```python
from build123d import *

# Parameters (mm, degrees)
SKETCH1_R                = 14.5
BOSS_EXTRUDE1_DEPTH      = 4
BOSS_EXTRUDE2_DEPTH      = 2
BOSS_EXTRUDE2_DEPTH_BACK = 125
SKETCH2_R                = 5
SKETCH2_R_2              = 4
SKETCH2_R_3              = 3.479997652
SKETCH2_R_4              = 2.479997652
LPATTERN4_START          = -124
LPATTERN4_OUTLINE_R      = 14.5
LPATTERN4_DEPTH          = 4
LPATTERN4_START_2        = -62
LPATTERN4_2_OUTLINE_R    = 14.5
LPATTERN4_2_OUTLINE_R_2  = 3.479997652
LPATTERN4_2_OUTLINE_R_3  = 5
LPATTERN4_2_OUTLINE_R_4  = 4
LPATTERN4_2_OUTLINE_R_5  = 2.479997652
LPATTERN4_2_DEPTH        = 4
SKETCH8_R                = 2.479997652
CUT_EXTRUDE4_DEPTH       = 128
SKETCH12_R               = 3.125
BOSS_EXTRUDE4_DEPTH      = 48
CUT_EXTRUDE5_DEPTH       = 48
SKETCH14_R               = 4
CUT_EXTRUDE6_DEPTH       = 124
SKETCH16_R               = 12.25
SKETCH16_R_2             = 2.479997652
BOSS_EXTRUDE5_DEPTH      = 7


# Read off the part's stored shape, not the designer's step: LPattern4
with BuildPart() as part:
    # Sketch1 → Boss-Extrude1 (new body)
    with BuildSketch(Plane(origin=(0, 0, 0), x_dir=(1, 0, 0), z_dir=(0, 1, 0))):
        with Locations(Location((0, 0, 0), (0, 0, 270))):
            Circle(SKETCH1_R)
    extrude(amount=BOSS_EXTRUDE1_DEPTH)

    # Sketch2 → Boss-Extrude2 (add, two sides: drawn at the far end of the back side and taken through both)
    # profile 1 of 7: a face of its own
    with BuildSketch(Plane(origin=(0, 4, 0), x_dir=(1, 0, 0), z_dir=(0, 1, 0)).offset(-BOSS_EXTRUDE2_DEPTH_BACK)):
        with Locations(Location((0, 0, 0), (0, 0, 270))):
            Circle(SKETCH2_R)
        with Locations(Location((0, 0, 0), (0, 0, 270))):
            Circle(SKETCH2_R_2, mode=Mode.SUBTRACT)
    # profile 2 of 7: a face of its own
    with BuildSketch(Plane(origin=(0, 4, 0), x_dir=(1, 0, 0), z_dir=(0, 1, 0)).offset(-BOSS_EXTRUDE2_DEPTH_BACK)):
        with Locations(Location((0, 9.5, 0), (0, 0, 270))):
            Circle(SKETCH2_R_3)
        with Locations(Location((0, 9.5, 0), (0, 0, 270))):
            Circle(SKETCH2_R_4, mode=Mode.SUBTRACT)
    # profile 3 of 7: a face of its own
    with BuildSketch(Plane(origin=(0, 4, 0), x_dir=(1, 0, 0), z_dir=(0, 1, 0)).offset(-BOSS_EXTRUDE2_DEPTH_BACK)):
        with Locations(Location((8.227241336, 4.75, 0), (0, 0, 270))):
            Circle(SKETCH2_R_3)
        with Locations(Location((8.227241336, 4.75, 0), (0, 0, 270))):
            Circle(SKETCH2_R_4, mode=Mode.SUBTRACT)
    # profile 4 of 7: a face of its own
    with BuildSketch(Plane(origin=(0, 4, 0), x_dir=(1, 0, 0), z_dir=(0, 1, 0)).offset(-BOSS_EXTRUDE2_DEPTH_BACK)):
        with Locations(Location((8.227241336, -4.75, 0), (0, 0, 270))):
            Circle(SKETCH2_R_3)
        with Locations(Location((8.227241336, -4.75, 0), (0, 0, 270))):
            Circle(SKETCH2_R_4, mode=Mode.SUBTRACT)
    # profile 5 of 7: a face of its own
    with BuildSketch(Plane(origin=(0, 4, 0), x_dir=(1, 0, 0), z_dir=(0, 1, 0)).offset(-BOSS_EXTRUDE2_DEPTH_BACK)):
        with Locations(Location((0, -9.5, 0), (0, 0, 270))):
            Circle(SKETCH2_R_3)
        with Locations(Location((0, -9.5, 0), (0, 0, 270))):
            Circle(SKETCH2_R_4, mode=Mode.SUBTRACT)
    # profile 6 of 7: a face of its own
    with BuildSketch(Plane(origin=(0, 4, 0), x_dir=(1, 0, 0), z_dir=(0, 1, 0)).offset(-BOSS_EXTRUDE2_DEPTH_BACK)):
        with Locations(Location((-8.227241336, -4.75, 0), (0, 0, 270))):
            Circle(SKETCH2_R_3)
        with Locations(Location((-8.227241336, -4.75, 0), (0, 0, 270))):
            Circle(SKETCH2_R_4, mode=Mode.SUBTRACT)
    # profile 7 of 7: a face of its own
    with BuildSketch(Plane(origin=(0, 4, 0), x_dir=(1, 0, 0), z_dir=(0, 1, 0)).offset(-BOSS_EXTRUDE2_DEPTH_BACK)):
        with Locations(Location((-8.227241336, 4.75, 0), (0, 0, 270))):
            Circle(SKETCH2_R_3)
        with Locations(Location((-8.227241336, 4.75, 0), (0, 0, 270))):
            Circle(SKETCH2_R_4, mode=Mode.SUBTRACT)
    extrude(amount=BOSS_EXTRUDE2_DEPTH + BOSS_EXTRUDE2_DEPTH_BACK)

    # LPattern4 outline → LPattern4 (add)
    with BuildSketch(Plane(origin=(0, 0, 0), x_dir=(1, 0, 0), z_dir=(0, 1, 0)).offset(LPATTERN4_START)):
        Circle(LPATTERN4_OUTLINE_R)
    extrude(amount=LPATTERN4_DEPTH)

    # LPattern4 2 outline → LPattern4 2 (add)
    # profile 1 of 8: a face of its own
    with BuildSketch(Plane(origin=(0, 0, 0), x_dir=(1, 0, 0), z_dir=(0, 1, 0)).offset(LPATTERN4_START_2)):
        Circle(LPATTERN4_2_OUTLINE_R)
        with Locations((-8.227241336, -4.75)):
            Circle(LPATTERN4_2_OUTLINE_R_2, mode=Mode.SUBTRACT)
        with Locations((0, -9.5)):
            Circle(LPATTERN4_2_OUTLINE_R_2, mode=Mode.SUBTRACT)
        with Locations((8.227241336, -4.75)):
            Circle(LPATTERN4_2_OUTLINE_R_2, mode=Mode.SUBTRACT)
        with Locations((-8.227241336, 4.75)):
            Circle(LPATTERN4_2_OUTLINE_R_2, mode=Mode.SUBTRACT)
        Circle(LPATTERN4_2_OUTLINE_R_3, mode=Mode.SUBTRACT)
        with Locations((8.227241336, 4.75)):
            Circle(LPATTERN4_2_OUTLINE_R_2, mode=Mode.SUBTRACT)
        with Locations((0, 9.5)):
            Circle(LPATTERN4_2_OUTLINE_R_2, mode=Mode.SUBTRACT)
    # profile 2 of 8: a face of its own
    with BuildSketch(Plane(origin=(0, 0, 0), x_dir=(1, 0, 0), z_dir=(0, 1, 0)).offset(LPATTERN4_START_2)):
        Circle(LPATTERN4_2_OUTLINE_R_4)
    # profile 3 of 8: a face of its own
    with BuildSketch(Plane(origin=(0, 0, 0), x_dir=(1, 0, 0), z_dir=(0, 1, 0)).offset(LPATTERN4_START_2)):
        with Locations((0, 9.5)):
            Circle(LPATTERN4_2_OUTLINE_R_5)
    # profile 4 of 8: a face of its own
    with BuildSketch(Plane(origin=(0, 0, 0), x_dir=(1, 0, 0), z_dir=(0, 1, 0)).offset(LPATTERN4_START_2)):
        with Locations((8.227241336, 4.75)):
            Circle(LPATTERN4_2_OUTLINE_R_5)
    # profile 5 of 8: a face of its own
    with BuildSketch(Plane(origin=(0, 0, 0), x_dir=(1, 0, 0), z_dir=(0, 1, 0)).offset(LPATTERN4_START_2)):
        with Locations((8.227241336, -4.75)):
            Circle(LPATTERN4_2_OUTLINE_R_5)
    # profile 6 of 8: a face of its own
    with BuildSketch(Plane(origin=(0, 0, 0), x_dir=(1, 0, 0), z_dir=(0, 1, 0)).offset(LPATTERN4_START_2)):
        with Locations((0, -9.5)):
            Circle(LPATTERN4_2_OUTLINE_R_5)
    # profile 7 of 8: a face of its own
    with BuildSketch(Plane(origin=(0, 0, 0), x_dir=(1, 0, 0), z_dir=(0, 1, 0)).offset(LPATTERN4_START_2)):
        with Locations((-8.227241336, -4.75)):
            Circle(LPATTERN4_2_OUTLINE_R_5)
    # profile 8 of 8: a face of its own
    with BuildSketch(Plane(origin=(0, 0, 0), x_dir=(1, 0, 0), z_dir=(0, 1, 0)).offset(LPATTERN4_START_2)):
        with Locations((-8.227241336, 4.75)):
            Circle(LPATTERN4_2_OUTLINE_R_5)
    extrude(amount=LPATTERN4_2_DEPTH)

    # Sketch8 → Cut-Extrude4 (cut)
    with BuildSketch(Plane(origin=(0, 4, 0), x_dir=(1, 0, 0), z_dir=(0, 1, 0))):
        with Locations(Location((-8.227241336, -4.75, 0), (0, 0, 270))):
            Circle(SKETCH8_R)
        with Locations(Location((0, -9.5, 0), (0, 0, 270))):
            Circle(SKETCH8_R)
        with Locations(Location((8.227241336, -4.75, 0), (0, 0, 270))):
            Circle(SKETCH8_R)
        with Locations(Location((8.227241336, 4.75, 0), (0, 0, 270))):
            Circle(SKETCH8_R)
        with Locations(Location((0, 9.5, 0), (0, 0, 270))):
            Circle(SKETCH8_R)
        with Locations(Location((-8.227241336, 4.75, 0), (0, 0, 270))):
            Circle(SKETCH8_R)
    extrude(amount=-CUT_EXTRUDE4_DEPTH, mode=Mode.SUBTRACT)

    # Sketch12 → Boss-Extrude4 (add)
    with BuildSketch(Plane.XZ.offset(124)):
        with Locations(Location((0, 0, 0), (0, 0, 90))):
            Circle(SKETCH12_R)
    extrude(amount=BOSS_EXTRUDE4_DEPTH)

    # Sketch9 → Cut-Extrude5 (cut)
    with BuildSketch(Plane.XZ.offset(172)):
        with BuildLine():
            Line((1.55, 1.489966443), (1.55, -1.489966443))
            ThreePointArc((1.55, -1.489966443), (-2.15, 0), (1.55, 1.489966443))
        make_face()
    extrude(amount=-CUT_EXTRUDE5_DEPTH, mode=Mode.SUBTRACT)

    # Sketch14 → Cut-Extrude6 (cut)
    with BuildSketch(Plane(origin=(0, 4, 0), x_dir=(1, 0, 0), z_dir=(0, 1, 0))):
        with Locations(Location((0, 0, 0), (0, 0, 270))):
            Circle(SKETCH14_R)
    extrude(amount=-CUT_EXTRUDE6_DEPTH, mode=Mode.SUBTRACT)

    # Sketch16 → Boss-Extrude5 (add)
    with BuildSketch(Plane.XZ.offset(124)):
        with Locations(Location((0, 0, 0), (0, 0, 90))):
            Circle(SKETCH16_R)
        with Locations(Location((0, 9.5, 0), (0, 0, 90))):
            Circle(SKETCH16_R_2, mode=Mode.SUBTRACT)
        with Locations(Location((8.227241336, 4.75, 0), (0, 0, 90))):
            Circle(SKETCH16_R_2, mode=Mode.SUBTRACT)
        with Locations(Location((8.227241336, -4.75, 0), (0, 0, 90))):
            Circle(SKETCH16_R_2, mode=Mode.SUBTRACT)
        with Locations(Location((0, -9.5, 0), (0, 0, 90))):
            Circle(SKETCH16_R_2, mode=Mode.SUBTRACT)
        with Locations(Location((-8.227241336, -4.75, 0), (0, 0, 90))):
            Circle(SKETCH16_R_2, mode=Mode.SUBTRACT)
        with Locations(Location((-8.227241336, 4.75, 0), (0, 0, 90))):
            Circle(SKETCH16_R_2, mode=Mode.SUBTRACT)
    extrude(amount=BOSS_EXTRUDE5_DEPTH)


solid = part.part
```
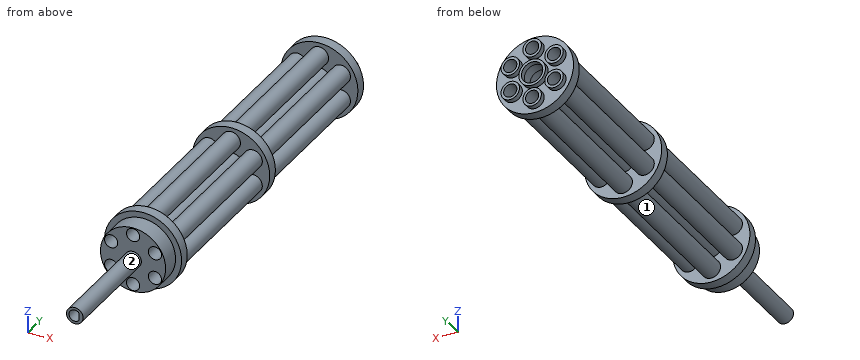
Here's how the part is built. I have some questions about the finished solid (model axes, mm). Face numbers are marked on the shaded views. Round coordinates to 2 decimals unless told otherwise and drop trailing zeros. Use CSV: the item, a comma, the result in double quotes.
1) If we mould it in two halves opening along Z, with no side actions, what happens to the marked faces 1 and 2? For each: pulls with the +Z half, pulls with the -Z half, needs draft (parallel to the pull), parting line crosses it, or undercut.
Taken from the geometry:
face 1,"undercut"
face 2,"parting line crosses it"
2) I'm going to push flat-ended pins straight in: P1, Ø8, axis at x = -8.23, z = 4.75, coming from the -Y side; P2, Ø3, axis at y = -12, z = -4, coming from the +X side; P3, Ø0.9, axis at y = -144.5, z = 0, coming from the -X side (3 decimals). Where does each tip first touch, or does it pass through?
Taken from the geometry:
P1,"y = -131"
P2,"x = 11.71"
P3,"x = -3.125"
3) I need wall thicknesses on line 1 along Y through (x, z) = (7.25, -10); line 2 along Y through (x, z) = (-9, -0.5); line 3 along Z through (x, y) = (8, -47.5). Which ranges of each line are inside material? Lowest first, please. Write a range as [from, to].
Taken from the geometry:
line 1,"[-124, -120], [-62, -58], [0, 4]"
line 2,"[-131, -120], [-62, -58], [0, 4]"
line 3,"[-8.22, -7.22], [-2.28, -1.28], [1.28, 2.28], [7.22, 8.22]"
4) I want a section at A-A (y = -103). Count the separate pieces of the cut face and the enclosed holes in it, then the cut area to 3 significant figures.
Taken from the geometry:
separate pieces,"7"
enclosed holes,"7"
area,"141 mm^2"
